from build123d import *

# Parameters (mm, degrees)
F2_R     = 2
F3_DEPTH = 25
F4_R     = 2
F5_DEPTH = 25


with BuildPart() as f1:
    # F0 (on Front) → F1 (revolve)
    with BuildSketch(Plane.XZ):
        Polygon((8, 8.6), (2.5, 8.6), (2.5, -7.4), (8, -7.4), (8, 0), (6, 0), (6, 7.2), (8, 7.2), align=None)
    revolve(axis=Axis((0, 0, 2.562595), (0, 0, -1)))

    # F2 (on Right) → F3 (cut)
    with BuildSketch(Plane.YZ):
        with Locations((0, -3.4)):
            Circle(F2_R)
    extrude(amount=F3_DEPTH, mode=Mode.SUBTRACT)

    # F4 (on Front) → F5 (cut)
    with BuildSketch(Plane.XZ):
        with Locations((0, -3.4)):
            Circle(F4_R)
    extrude(amount=-F5_DEPTH, mode=Mode.SUBTRACT)


solid = f1.part
Input: part model. Units: mm. Frame: model coordinates. A direction names the side the tool comes from. Give positions to 0.01 mm unless a question says otherwise; leave off trailing zeros. Write each loop counter-clockwise with the first axis right and the second up, starting at its lowest first coordinate (ties: lowest second). Pieces come first, ordered by that corner, then holes. Notation, with made-up numbers: M 59,44.5 L 72,44.5 A28 cw 72,78.5 Z; hole C 71,-30.5 d8. An arc over 180 degrees is marked long. Write item = value, one per line. Start each with the question number.
1) Cut plane C-C on z = -1.75. Return the cut outline in (x, y).
2) Material intervals for line 1 along Z through (x, y) = (0, 6.75); line 2 along X through (y, z) = (0, -1); line 3 along X through (y, z) = (0, 4), sorted ascending. Write a range as [from, to].
3) Cut plane A-A on y = 0. Return the cut outline in (x, z), then the cut area to 3 significant figures.
4) Cut plane D-D on y = -6.5. Return the cut outline in (x, z).
5) Reachability of faces 1 (the cylindrical face through (4.301, -6.746, -3.648)), 2 (the cylindrical face through (-1.998, 4.708, -3.312)), 3 (the cylindrical face through (-6, 0, 4)) from +Z, -Z, +X, -X, +Y, -Y: full face, straight path, thin tool, end or side. Return the list, or none.
6) First-contact query: pin 1 Ø2 at (y, z) = (-2.5, 1.5) entering from -X; pin 2 Ø8 at (x, z) = (4.5, -5) entering from +Y; pin 3 Ø1 at (y, z) = (4, -5.5) entering from +X. Flat tips, straight axial feed; report the tip coordinate or a pass-through.
7) Draft query along Z for faces 4 (the flat face through (2, 2, -7.4)), 5 (the cylindrical face through (-1.73, 7.81, 7.91)), 6 (the cylindrical face through (4.704, -1.998, -3.312)), 7 (the flat face through (-2, 2, 8.6)). Return one class per face: +Z half, -Z half, draft (parallel to the pull), parting line (faces both ways), or undercut.
Solved:
q1.outline = M -1.13,2.23 L -1.13,7.92 A8 ccw long 7.92,-1.13 L 2.23,-1.13 A2.5 cw long Z; M 1.13,2.23 A2.5 cw 2.23,1.13 L 7.92,1.13 A8 ccw 1.13,7.92 Z
q2.line_1 = [-7.4, -5.4], [-1.4, 0], [7.2, 8.6]
q2.line_2 = [-8, -2.5], [2.5, 8]
q2.line_3 = [-6, -2.5], [2.5, 6]
q3.outline = M -8,-7.4 L -2.5,-7.4 L -2.5,8.6 L -8,8.6 L -8,7.2 L -6,7.2 L -6,0 L -8,0 Z; M 2.5,-7.4 L 8,-7.4 L 8,-5.4 L 2.5,-5.4 Z; M 2.5,-1.4 L 8,-1.4 L 8,0 L 6,0 L 6,7.2 L 8,7.2 L 8,8.6 L 2.5,8.6 Z
q3.area = 125 mm2
q4.outline = M -4.66,-7.4 L 4.66,-7.4 L 4.66,0 L -4.66,0 Z; M -4.66,7.2 L 4.66,7.2 L 4.66,8.6 L -4.66,8.6 Z
q5.face_1 = +Z, -Z
q5.face_2 = +Y
q5.face_3 = none
q6.pin_1 = -5.81
q6.pin_2 = 7.98
q6.pin_3 = 7.19
q7.face_4 = -Z half
q7.face_5 = draft
q7.face_6 = undercut
q7.face_7 = +Z half
